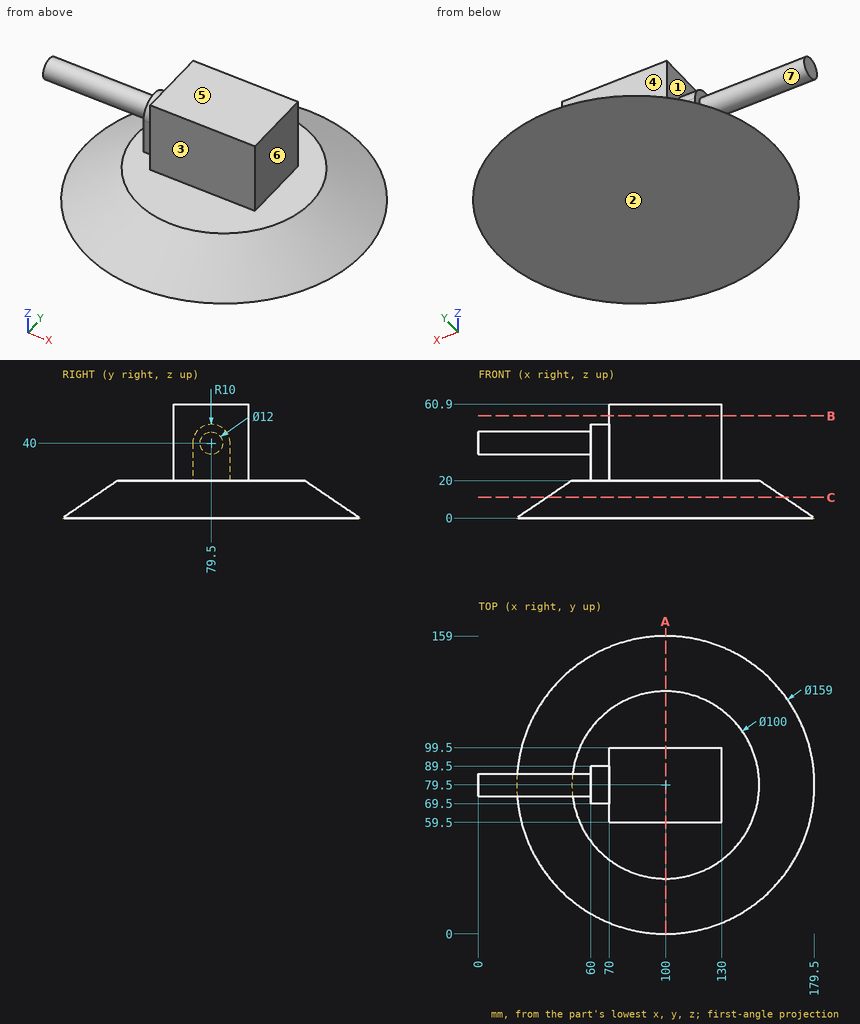
Source: three-view drawing plus pictorial views. Frame: mm from the lowest corner of the part. A direction names the side the tool comes from. Round coordinates to 2 decimals unless told otherwise and drop trailing zeros. Loops run counter-clockwise (first coordinate to the right, second up) from the corner with the lowest first, then second, coordinate; pieces in that order, holes last. Notation, with made-up numbers: M 11.5,89 L 31.5,89 A22 ccw 31.5,102 Z; hole C 60,66.25 d4. An arc over 180 degrees is marked long. Put each result on its own line as item: value. Start each with the question number.
(1) Section query C-C (z = 11). Return loops of the section in (x, y) (3 decimals).
(2) Section query B-B (z = 54.5). Return loops of the section in (x, y).
(3) Draft query along Z for the marked faces 5, 6 and 7. Return one class per face: +Z half, -Z half, draft (parallel to the pull), parting line (faces both ways), or undercut.
(4) Contact query for flat-ended pins moving along their axis: pin 1 Ø1 at (y, z) = (79.5, 14.5) entering from -X; pin 2 Ø20.5 at (x, z) = (105, 34.5) entering from +Y; pin 3 Ø8 at (x, z) = (65.5, 26) entering from -Y; pin 4 Ø22 at (y, z) = (75, 34.5) entering from -X. Output: stop coordinate, or through.
(5) Section query A-A (x = 100). Return loops of the section in (y, z), then the cut area to 3 significant figures.
(6) Material intervals for line 1 along Z through (x, y) = (105, 33); line 2 along X through (y, z) = (63.5, 22.5); line 3 along Y through (x, z) = (96, 49.5), sorted ascending. Write a range as [from, to].
(7) Set-up query: the marked faces 1, 2, 3 and 4. Return all of +Z, -Z, +X, -X, +Y, -Y with unobstructed straight access to the full face (end or side cutting, diameter ignored); none if empty.
Findings below:
1. outline: C 100,79.5 d126.55
2. outline: M 70,59.5 L 130,59.5 L 130,99.5 L 70,99.5 Z
3. face 5: +Z half
3. face 6: draft
3. face 7: undercut
4. pin 1: stops at x = 41.15
4. pin 2: stops at y = 99.5
4. pin 3: stops at y = 69.5
4. pin 4: stops at x = 0
5. outline: M 0,0 L 159,0 L 129.5,20 L 99.5,20 L 99.5,60.9 L 59.5,60.9 L 59.5,20 L 29.5,20 Z
5. area: 4,230 mm2
6. line 1: z = [0, 20]
6. line 2: x = [70, 130]
6. line 3: y = [59.5, 99.5]
7. face 1: +Z, -X
7. face 2: -Z, +X, -X, +Y, -Y
7. face 3: +Z, +X, -X, -Y
7. face 4: +Z, +X, -X, +Y
